Print and shaded views of the part. All mm, measured from the part's lowest x, y and z. A direction names the side the tool comes from. Round coordinates to 2 decimals unless told otherwise and drop trailing zeros. Loops run counter-clockwise (first coordinate to the right, second up) from the corner with the lowest first, then second, coordinate; pieces in that order, holes last. Notation, with made-up numbers: M 46,21.25 L 92,21.25 A21 cw 92,58.25 Z; hole C -24.75,-1.5 d1. An arc over 180 degrees is marked long. One line per item, written item: value. Start each with the question number.
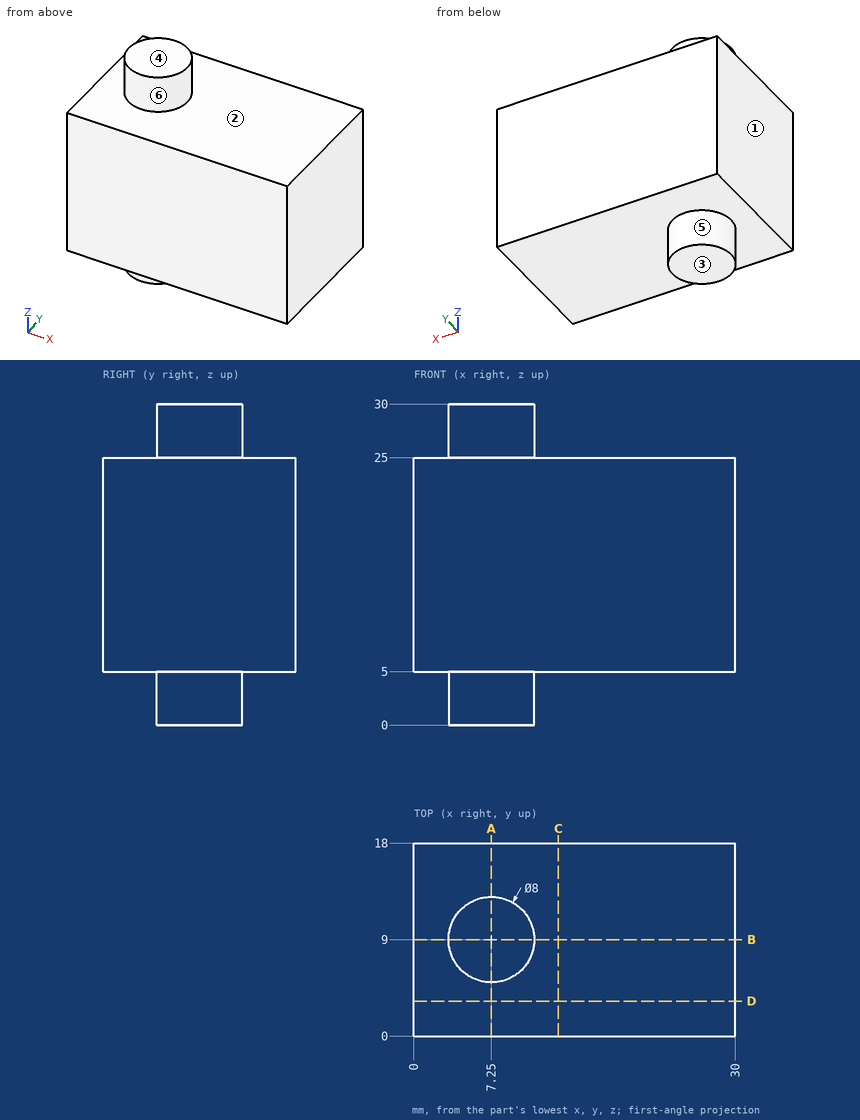
(1) Slice it at A-A, the plane x = 7.25. List the corners of the cut face in (y, z).
(2) Flat gauge pin, fed straight in: P1, Ø1.5, axis at x = 13, y = 3.5, coming from the -Z side. Where does the tip first touch, or does it go through?
(3) Probe L1, parallel to Z at x = 3.5, y = 11.25; L2, parallel to X at y = 10, z = 27.75; L3, parallel to Y at x = 9, z = 1.5. List the from-to ranges inside material, lowest first.
(4) Slice it at D-D, the plane y = 3.25. List the corners of the cut face in (x, z).
(5) Slice it at C-C, the plane x = 13.5. List the corners of the cut face in (y, z), and give its area (3 significant figures).
(6) Slice it at B-B, the plane y = 9. List the corners of the cut face in (x, z), and give its area (3 significant figures).
(7) Which spindle directions (+Z, -Z, +X, -X, +Y, -Y) get a long thin tool onto all of the face, cutting with end or side? Do the marked faces 4, 5 and 6. Say none if no direction does.
(8) Mould opens along Z. For the marked faces 1, 2 and 3 say: pulls with the +Z half, pulls with the -Z half, needs draft (parallel to the pull), parting line crosses it, or undercut.
Check result:
1. outline: M 0,5 L 5,5 L 5,0 L 13,0 L 13,5 L 18,5 L 18,25 L 13,25 L 13,30 L 5,30 L 5,25 L 0,25 Z
2. P1: stops at z = 5
3. L1: z = 5 to 25
3. L2: x = 3.38 to 11.12
3. L3: y = 5.4 to 12.6
4. outline: M 0,5 L 30,5 L 30,25 L 0,25 Z
5. outline: M 0,5 L 18,5 L 18,25 L 0,25 Z
5. area: 360 mm^2
6. outline: M 0,5 L 3.25,5 L 3.25,0 L 11.25,0 L 11.25,5 L 30,5 L 30,25 L 11.25,25 L 11.25,30 L 3.25,30 L 3.25,25 L 0,25 Z
6. area: 680 mm^2
7. face 4: +Z, +X, -X, +Y, -Y
7. face 5: -Z
7. face 6: +Z
8. face 1: needs draft
8. face 2: pulls with the +Z half
8. face 3: pulls with the -Z half
